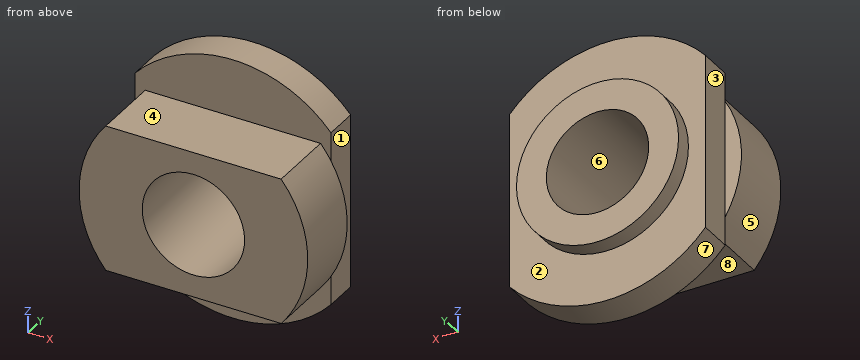
Autodesk Inventor part; units mm, degrees
ref_plane "YZ Plane" through (0, 0, 0) normal (1, 0, 0) x (0, 1, 0)
ref_plane "XZ Plane" through (0, 0, 0) normal (0, 1, 0) x (-1, 0, 0)
ref_plane "XY Plane" through (0, 0, 0) normal (0, 0, 1) x (1, 0, 0)
sketch "Sketch1" plane through (0, 0, 0) normal (0, 0, 1) x (1, 0, 0)
  line L0 (0, 0) -> (3.35, 0)
  line L1 (3.35, 0) -> (3.35, 2)
  line L2 (3.35, 2) -> (0, 2)
  line L3 (0, 2) -> (0, 0)
  line L4 (0, 2) -> (3.85, 2)
  line L5 (3.85, 2) -> (3.85, 3)
  line L6 (3.85, 3) -> (0, 3)
  line L7 (0, 3) -> (0, 2)
  line L8 (0, 3) -> (2.375, 3)
  line L9 (2.375, 3) -> (2.375, 3.5)
  line L10 (2.375, 3.5) -> (0, 3.5)
  line L11 (0, 3.5) -> (0, 3)
  dimension "d0" = 6.7
  dimension "d1" = 7.7
  dimension "d2" = 4.75
  dimension "d3" = 2
  dimension "d4" = 3
  dimension "d5" = 3.5
revolve "Revolution1" add sketch "Sketch1" angle 360 about axis through (0, 3.5, 0) along (0, -1, 0)
sketch "Sketch2" plane through (0, 3, 0) normal (0, 1, 0) x (1, 0, 0)
  circle A0 centre (0, 0) radius 3.85
  line L0 (-2.875, 2.5606) -> (-2.875, -2.5606)
  line L1 (2.875, 2.5606) -> (2.875, -2.5606)
  dimension "d7" = 5.75
extrude "Extrusion1" cut sketch "Sketch2" against normal up to surface (1 mm away) contours A0 L1 | L0 A0
hole "Hole1" at (0, 3.5, 0) direction (0, -1, 0) diameter 3 end through all
sketch "Sketch3" plane through (0, 0, 0) normal (0, -1, 0) x (1, 0, 0)
  circle A0 centre (0, 0) radius 3.35
  line L0 (4, 2.15) -> (4, 4.15)
  line L1 (4, 4.15) -> (-4, 4.15)
  line L2 (-4, 4.15) -> (-4, 2.15)
  line L3 (-4, 2.15) -> (4, 2.15)
  line L4 (4, -2.15) -> (4, -4.15)
  line L5 (4, -4.15) -> (-4, -4.15)
  line L6 (-4, -4.15) -> (-4, -2.15)
  line L7 (-4, -2.15) -> (4, -2.15)
  line L8 (0, 2.15) -> (0, -2.15) construction
  point P0 (0, 0)
  dimension "d19" = 4.3
  dimension "d20" = 2
  dimension "d21" = 8
extrude "Extrusion2" cut sketch "Sketch3" against normal up to surface (2 mm away) contours L3 A0 | A0 L3 L2 L1 L0 | L7 L4 L5 L6 A0 | A0 L7
properties part number "308-08" material "Polypropylene"
For this review, take the finished solid that the model builds, in its own axes (mm). Face numbers are marked on the shaded views. A direction names the side the tool comes from. Give positions to 0.01 mm unless a question says otherwise; leave off trailing zeros. Order: outer loops, then holes, each group sorted by start corner. A loop starts at its lowest first (then second) coordinate and runs counter-clockwise, first axis right, second up. Notation, with made-up numbers: (31, 22.5) -> (85, 22.5) arc R23 cw to (85, 42.5) -> close; hole circle Ø2 at (78.5, 53). An arc over 180 degrees is marked (long way). Write item = value, one per line.
1) We need section D-D, the plane z = 2.25. Give the boundary of the cut face in (x, y) (3 decimals).
Findings:
outline = (-2.875, 2) -> (2.875, 2) -> (2.875, 3) -> (0.76, 3) -> (0.76, 3.5) -> (-0.76, 3.5) -> (-0.76, 3) -> (-2.875, 3) -> close
2) To check wall thickness, follow L1, parallel to Z at x = 0, y = 2.05; L2, parallel to X at y = 1.8, z = 0; L3, parallel to Z at x = 0, y = 1.5. State the ranges of each line that lie inside material, in increasing order. Write a range as from..to.
Findings:
L1 = -3.85..-1.5, 1.5..3.85
L2 = -3.35..-1.5, 1.5..3.35
L3 = -2.15..-1.5, 1.5..2.15
3) We need section C-C, the plane y = 1.15. Give the boundary of the cut face in (x, z), and give its area (3 significant figures).
Findings:
outline = (-2.57, -2.15) -> (2.57, -2.15) arc R3.35 ccw to (2.57, 2.15) -> (-2.57, 2.15) arc R3.35 ccw to start; hole circle Ø3 at (0, 0)
area = 19.6 mm^2
4) Insertion check: pin 1 (1 mm diameter, centred on x = 0.5, y = 1, fed in from -Z); pin 2 (1 mm diameter, centred on y = 1, z = 1.5, fed in from +X); pin 3 (2.5 mm diameter, centred on x = -1.5, z = -3, fed in from -Y); pin 4 (0.5 mm diameter, centred on x = -3, z = 0.5, fed in from +Y). Each pin has a flat end and moves straight along its axis. Give the tip position at first contact, or say it passes through.
Findings:
pin_1 = -2.15
pin_2 = 3.2
pin_3 = 0
pin_4 = 3
5) For the marked faces 1, 2, 3, 4 and 5, list the 3-axis set-ups (+Z, -Z, +X, -X, +Y, -Y) from which the entire face can be reached by the end or side of a thin tool; tool diameter is ignored.
Findings:
face_1 = +Z, -Z, +X, +Y
face_2 = +Y
face_3 = +Z, -Z, -X, +Y
face_4 = +Z, +X, -X, -Y
face_5 = -X, -Y
6) We need section A-A, the plane x = 0. Give the boundary of the cut face in (y, z) (3 decimals), and give its area (4 significant figures).
Findings:
outline = (0, -2.15) -> (2, -2.15) -> (2, -3.85) -> (3, -3.85) -> (3, -2.375) -> (3.5, -2.375) -> (3.5, -1.5) -> (0, -1.5) -> close; (0, 1.5) -> (3.5, 1.5) -> (3.5, 2.375) -> (3, 2.375) -> (3, 3.85) -> (2, 3.85) -> (2, 2.15) -> (0, 2.15) -> close
area = 8.175 mm^2
7) We need section B-B, the plane z = 0.5. Give the boundary of the cut face in (x, y) (3 decimals).
Findings:
outline = (-3.312, 0) -> (-1.414, 0) -> (-1.414, 3.5) -> (-2.322, 3.5) -> (-2.322, 3) -> (-2.875, 3) -> (-2.875, 2) -> (-3.312, 2) -> close; (1.414, 0) -> (3.312, 0) -> (3.312, 2) -> (2.875, 2) -> (2.875, 3) -> (2.322, 3) -> (2.322, 3.5) -> (1.414, 3.5) -> close
8) Draft analysis for pull direction X (two halves, no side actions). For the marked faces 6, 7 and 8, state which applies: pulls with the +X half, pulls with the -X half, needs draft (parallel to the pull), parting line crosses it, or undercut.
Findings:
face_6 = undercut
face_7 = parting line crosses it
face_8 = needs draft
